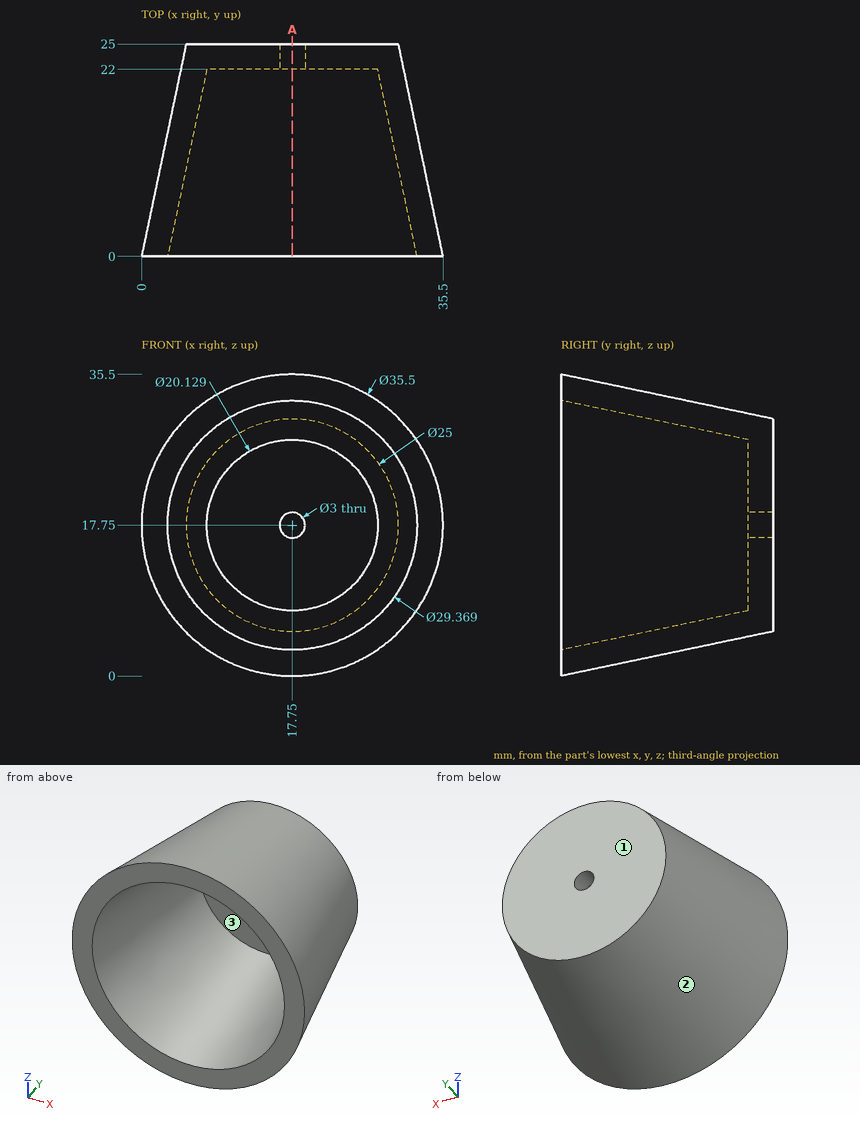
Part print with two shaded views. Sizes in mm from the minimum x, y, z corner. Coordinates: 2 decimals unless noted, no trailing zeros. Write each loop counter-clockwise with the first axis right and the second up, starting at its lowest first coordinate (ties: lowest second). Pieces come first, ordered by that corner, then holes. Notation, with made-up numbers: (0.5, 6) -> (46.5, 6) arc R9 cw to (46.5, 22) -> close; hole circle Ø8 at (-38.5, -33). An arc over 180 degrees is marked (long way). Return JSON: item names as keys, results as strings. Group by question number.
Q1. Pull direction Z, two halves, no side cores. Call the marked faces 1, 2 and 3: released by +Z, released by -Z, zero draft, split by the parting line, or undercut.
Q2. Flat gauge pins, fed straight in: pin 1 (5 mm diameter, centred on y = 11.5, z = 28, fed in from -X); pin 2 (5 mm diameter, centred on x = 31, y = 8, fed in from -Z); pin 3 (5 mm diameter, centred on x = 18.5, y = 14.5, fed in from +Z). Where does each tip first touch, or does it go through?
Q3. Cut at A-A, the plane x = 17.75. Give the cut face in (y, z), then the cut area to 3 significant figures.
Q4. Drill centre lines: line 1 (Y direction, x = 18.5, z = 15); line 2 (X direction, y = 14.5, z = 9.5); line 3 (X direction, y = 4, z = 15) (1 decimal). Where is each one in solid material? Low to high.
Returned:
{
 "1": {"face 1": "zero draft", "face 2": "split by the parting line", "face 3": "undercut"},
 "2": {"pin 1": "stops at x = 4.4", "pin 2": "stops at z = 5.7", "pin 3": "stops at z = 32.97"},
 "3": {"outline": "(0, 0) -> (25, 5.25) -> (25, 16.25) -> (22, 16.25) -> (22, 7.69) -> (0, 3.07) -> close; (0, 32.43) -> (22, 27.81) -> (22, 19.25) -> (25, 19.25) -> (25, 30.25) -> (0, 35.5) -> close", "area": "203 mm2"},
 "4": {"line 1": "y = 22 to 25", "line 2": "x = 5.58 to 9.54, 25.96 to 29.92", "line 3": "x = 1.1 to 4.2, 31.3 to 34.4"}
}
